Verification items for the finished model (mm, model axes). Coordinates: 2 decimals unless noted, no trailing zeros. Loops run counter-clockwise (first coordinate to the right, second up) from the corner with the lowest first, then second, coordinate; pieces in that order, holes last. Notation, with made-up numbers: (69, 82) -> (92, 82) arc R9 ccw to (92, 99) -> close; hole circle Ø6 at (15, 22). An arc over 180 degrees is marked (long way). Answer as a JSON object with one key per item and string values. Group by question number.
Q1. Cross-section at A-A on x = 42. Record the boundary of the cut face in (y, z), and give its area (3 significant figures).
Q2. Gauge pin test, flat ends, axial feed: pin 1 Ø4.5 at (x, y) = (109.5, 96.75) entering from -Z; pin 2 Ø1.2 at (x, z) = (-28.5, 0.5) entering from -Y. Record the tip position at first contact, or that the pin passes through.
Q3. Scan lines: L1, parallel to X at y = -70.25, z = 1; L2, parallel to Y at x = 109.5, z = 0.6; L3, parallel to Y at x = -140, z = 0.05. Record each from-to range of solid material in increasing order.
Q4. Cross-section at B-B on z = -1.25. Give the number of separate pieces and of enclosed holes in the cut face, and give its area (3 significant figures).
Q5. Cross-section at C-C on y = 64. Record the boundary of the cut face in (x, z).
Autodesk Inventor part; units mm, degrees
ref_plane "YZ Plane" through (0, 0, 0) normal (1, 0, 0) x (0, 1, 0)
ref_plane "XZ Plane" through (0, 0, 0) normal (0, 1, 0) x (-1, 0, 0)
ref_plane "XY Plane" through (0, 0, 0) normal (0, 0, 1) x (1, 0, 0)
sketch "Hinges" plane through (0, 0, 0) normal (0, 0, 1) x (1, 0, 0)
  circle A0 centre (-464.8647, 95.9101) radius 1.75
  circle A1 centre (-464.8647, 121.4101) radius 1.75
  line L0 (-471.3647, 88.6601) -> (-455.3647, 88.6601)
  line L1 (-455.3647, 88.6601) -> (-455.3647, 128.6601)
  line L2 (-455.3647, 128.6601) -> (-471.3647, 128.6601)
  line L3 (-471.3647, 128.6601) -> (-471.3647, 88.6601)
  circle A2 centre (-439.8647, 121.4101) radius 1.75
  circle A3 centre (-439.8647, 95.9101) radius 1.75
  line L4 (-433.3647, 128.6601) -> (-449.3647, 128.6601)
  line L5 (-449.3647, 128.6601) -> (-449.3647, 88.6601)
  line L6 (-449.3647, 88.6601) -> (-433.3647, 88.6601)
  line L7 (-433.3647, 88.6601) -> (-433.3647, 128.6601)
  point P0 (-452.3647, 108.6601)
  dimension "d30" = 3.5
  dimension "d31" = 25.5
  dimension "d32" = 6.5
  dimension "d33" = 40
  dimension "d34" = 7.25
  dimension "d35" = 16
  dimension "d36" = 3.5
  dimension "d37" = 25.5
  dimension "d38" = 6.5
  dimension "d39" = 40
  dimension "d40" = 7.25
  dimension "d41" = 16
  dimension "d42" = 38
sketch "Sketch1" plane through (0, 0, 0) normal (0, 0, 1) x (1, 0, 0)
  line L0 (-148, 181) -> (148, 181)
  line L1 (148, 181) -> (148, -181)
  line L2 (148, -181) -> (-148, -181)
  line L3 (-148, -181) -> (-148, 181)
  line L4 (-75, -181) -> (-65, -171)
  line L5 (-75, -181) -> (-60.8579, -181) construction
  line L6 (-65, -171) -> (65, -171)
  line L7 (65, -171) -> (75, -181)
  line L8 (-125, -181) -> (-148, -158)
  line L9 (-125, -181) -> (-92.4731, -181) construction
  line L10 (125, -181) -> (148, -158)
  line L11 (125, -181) -> (157.5269, -181) construction
  line L12 (-148, 161) -> (-128, 181)
  line L13 (-148, 161) -> (-119.7157, 161) construction
  line L14 (148, 161) -> (128, 181)
  line L15 (-100, 134) -> (100, 134)
  line L16 (100, 134) -> (100, -133)
  line L17 (100, -133) -> (-100, -133)
  line L18 (-100, -133) -> (-100, 134)
  point P0 (0, 0)
  point P1 (0, 181)
  point P2 (-148, 0)
  point P3 (0, -171)
  point P4 (0, 134)
  dimension "d0" = 296
  dimension "d1" = 362
  dimension "d2" = 45
  dimension "d3" = 10
  dimension "d4" = 150
  dimension "d5" = 135
  dimension "d6" = 50
  dimension "d7" = 45
  dimension "d8" = 50
  dimension "d9" = 45
  dimension "d10" = 20
  dimension "d11" = 20
  dimension "d12" = 135
  dimension "d13" = 47
  dimension "d14" = 200
  dimension "d15" = 267
extrude "Extrusion1" add sketch "Sketch1" along normal mid plane 4 contours L0 L14 L1 L10 L2 L7 L6 L4 L8 L3 L12
chamfer "Chamfer1" distance 20 angle 45 4 edges at (-100, 134, 0) (100, 134, 0) (-100, -133, 0) (100, -133, 0)
sketch "Sketch3" plane through (0, 0, -2) normal (0, 0, -1) x (-1, 0, 0)
  circle A0 centre (-140, 150) radius 3
  circle A1 centre (-140, -150) radius 3
  circle A2 centre (140, -150) radius 3
  circle A3 centre (140, 150) radius 3
  line L0 (-148, 161) -> (-148, -158)
  line L1 (148, -158) -> (148, 161)
  point P0 (0, 0)
  dimension "d25" = 6
  dimension "d26" = 300
  dimension "d27" = 150
  dimension "d47" = 8
  dimension "d48" = 8
extrude "Extrusion3" cut sketch "Sketch3" against normal blind 37.5
sketch "Sketch4" plane through (0, 0, -2) normal (0, 0, -1) x (-1, 0, 0)
  line L0 (-100, -113) -> (-100, 114)
  line L1 (100, 114) -> (100, -113)
  circle A0 centre (-109.5, 71.25) radius 1.75
  circle A1 centre (-109.5, 96.75) radius 1.75
  line L2 (-116, 64) -> (-100, 64)
  line L3 (-100, 64) -> (-100, 104)
  line L4 (-100, 104) -> (-116, 104)
  line L5 (-116, 104) -> (-116, 64)
  circle A2 centre (-84.5, 96.75) radius 1.75
  circle A3 centre (-84.5, 71.25) radius 1.75
  line L6 (-78, 104) -> (-94, 104)
  line L7 (-94, 104) -> (-94, 64)
  line L8 (-94, 64) -> (-78, 64)
  line L9 (-78, 64) -> (-78, 104)
  circle A4 centre (-109.5, -95.75) radius 1.75
  circle A5 centre (-109.5, -70.25) radius 1.75
  line L10 (-116, -103) -> (-100, -103)
  line L11 (-100, -103) -> (-100, -63)
  line L12 (-100, -63) -> (-116, -63)
  line L13 (-116, -63) -> (-116, -103)
  circle A6 centre (-84.5, -70.25) radius 1.75
  circle A7 centre (-84.5, -95.75) radius 1.75
  line L14 (-78, -63) -> (-94, -63)
  line L15 (-94, -63) -> (-94, -103)
  line L16 (-94, -103) -> (-78, -103)
  line L17 (-78, -103) -> (-78, -63)
  circle A8 centre (84.5, -12.75) radius 1.75
  circle A9 centre (84.5, 12.75) radius 1.75
  line L18 (78, -20) -> (94, -20)
  line L19 (94, -20) -> (94, 20)
  line L20 (94, 20) -> (78, 20)
  line L21 (78, 20) -> (78, -20)
  circle A10 centre (109.5, 12.75) radius 1.75
  circle A11 centre (109.5, -12.75) radius 1.75
  line L22 (116, 20) -> (100, 20)
  line L23 (100, 20) -> (100, -20)
  line L24 (100, -20) -> (116, -20)
  line L25 (116, -20) -> (116, 20)
  point P0 (0, 0)
  point P1 (100, 0)
  dimension "d43" = 10
  dimension "d44" = 10
extrude "Extrusion4" cut sketch "Sketch4" against normal blind 10 contours A0 | A1 | A4 | A5 | A10 | A11
equation "\"d34\" = -0.5 * d31 + 0.5 * d33"
equation "\"d40\" = -0.5 * d37 + 0.5 * d39"
equation "\"d8\" = d6"
properties part number "Right Sides Cover" material "Wood (Birch)"
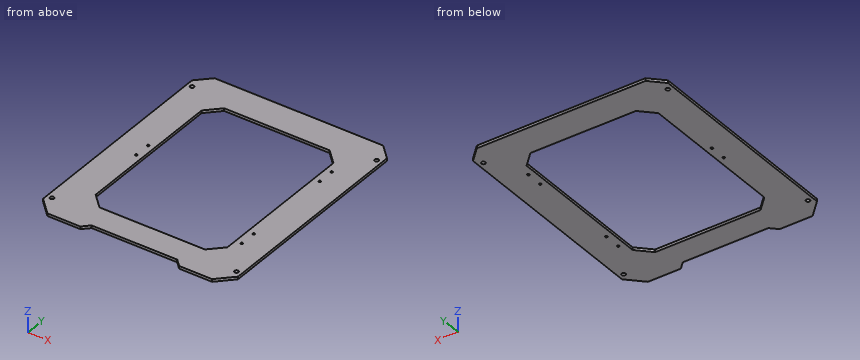
Computed values:
{
 "1": {"outline": "(-171, -2) -> (-133, -2) -> (-133, 2) -> (-171, 2) -> close; (134, -2) -> (181, -2) -> (181, 2) -> (134, 2) -> close", "area": "340 mm²"},
 "2": {"pin 1": "stops at z = -2", "pin 2": "stops at y = -171"},
 "3": {"L1": "x = -148 to -100, 100 to 107.75, 111.25 to 148", "L2": "y = -181 to -97.5, -94 to -72, -68.5 to 69.5, 73 to 95, 98.5 to 181", "L3": "y = -166 to -153, -147 to 147, 153 to 169"},
 "4": {"separate pieces": "1", "enclosed holes": "11", "area": "52,100 mm²"},
 "5": {"outline": "(-148, -2) -> (-100, -2) -> (-100, 2) -> (-148, 2) -> close; (100, -2) -> (148, -2) -> (148, 2) -> (100, 2) -> close"}
}
